from build123d import *

# Parameters (mm, degrees)
CUT_EXTRUDE1_DEPTH = 5
CUT_EXTRUDE2_DEPTH = 5


with BuildPart() as part:
    # Sketch1 → Revolve1 (revolve)
    with BuildSketch(Plane.XY, mode=Mode.PRIVATE) as revolve1_sk:
        Polygon((0, 0), (326, 0), (326, 16.5), (325, 17.5), (324, 17.5), (324, 16.1), (322.5, 16.1), (322.5, 17.5), (308.5, 17.5), (308.5, 20.5), (199.5, 20.5), (199.5, 17.5), (101.5, 17.5), (101.5, 16.1), (100, 16.1), (100, 17.5), (1, 17.5), (0, 16.5), align=None)
    revolve(revolve1_sk.sketch.rotate(Axis((0, 0, 0), (1, 0, 0)), 90), axis=Axis((0, 0, 0), (1, 0, 0)))

    # Sketch2 → Cut-Extrude1 (cut)
    with BuildSketch(Plane(origin=(0, 17.5, 0), x_dir=(1, 0, 0), z_dir=(0, 1, 0))):
        with BuildLine():
            Line((189.5, -5), (149.5, -5))
            ThreePointArc((149.5, -5), (144.5, 0), (149.5, 5))
            Line((149.5, 5), (189.5, 5))
            ThreePointArc((189.5, 5), (194.5, 0), (189.5, -5))
        make_face()
    extrude(amount=-CUT_EXTRUDE1_DEPTH, mode=Mode.SUBTRACT)

    # Sketch3 → Cut-Extrude2 (cut)
    with BuildSketch(Plane(origin=(0, 17.5, 0), x_dir=(1, 0, 0), z_dir=(0, 1, 0))):
        with BuildLine():
            Line((189.5, 5), (149.5, 5))
            ThreePointArc((149.5, 5), (144.5, 0), (149.5, -5))
            Line((149.5, -5), (189.5, -5))
            ThreePointArc((189.5, -5), (194.5, 0), (189.5, 5))
        make_face()
        with BuildLine():
            Line((10, 5), (50, 5))
            ThreePointArc((50, 5), (55, 0), (50, -5))
            Line((50, -5), (10, -5))
            ThreePointArc((10, -5), (5, 0), (10, 5))
        make_face()
    extrude(amount=-CUT_EXTRUDE2_DEPTH, mode=Mode.SUBTRACT)


solid = part.part
Verification items for the finished model (mm, model axes). A direction names the side the tool comes from. Round coordinates to 2 decimals unless told otherwise and drop trailing zeros. Loops run counter-clockwise (first coordinate to the right, second up) from the corner with the lowest first, then second, coordinate; pieces in that order, holes last. Notation, with made-up numbers: (54, -1.75) - (78, -1.75) arc R7 ccw to (78, 6.25) - close; hole circle Ø2 at (-5.75, -20.75). An arc over 180 degrees is marked (long way). Write item = value, one per line.
Q1. Material ranges on L1, parallel to X at y = -5.5, z = -16; L2, parallel to X at y = -12.5, z = 11; L3, parallel to X at y = -9.5, z = 15, recorded low to high.
Here are the results:
L1 = 0.42 to 100, 101.5 to 322.5, 324 to 325.58
L2 = 0.15 to 100, 101.5 to 322.5, 324 to 325.85
L3 = 199.5 to 308.5
Q2. Sectioned sample at D-D on x = 210. Record the boundary of the cut face in (y, z), plus the area to 3 significant figures.
Here are the results:
outline = circle Ø41 at (0, 0)
area = 1,320 mm^2
Q3. Depth check by flat-ended pin: pin 1 (4.5 mm diameter, centred on x = 37, y = 15, fed in from -Z); pin 2 (12 mm diameter, centred on x = 84, y = 4, fed in from -Z); pin 3 (3.5 mm diameter, centred on x = 38, y = 13.5, fed in from +Z); pin 4 (1 mm diameter, centred on y = 15.5, z = 0.5, fed in from -X). Enter the tip coordinate at first touch or a pass-through.
Here are the results:
pin_1 = -11.99
pin_2 = -17.5
pin_3 = 12.97
pin_4 = 0
Q4. Tool access check on faces 4 (the cylindrical face through (149.814, -14.756, 9.408)), 5 (the flat face through (322.5, 5.1, -15.5)), 6 (the flat face through (170, 12.5, 0)). Record the directions out of +Z, -Z, +X, -X, +Y, -Y that give a thin tool (end or side, any length) a straight path to the whole face; none if there is none.
Here are the results:
face_4 = -X
face_5 = none
face_6 = +Y
Q5. Mould release check, pull along X, two halves, no side actions. Record for faces 1 (the flat face through (199.5, -9.2, 15.1)), 2 (the flat face through (308.5, -9.2, -15.1)), 3 (the cylindrical face through (100.74, -4.836, 15.357)): +X half, -X half, draft (parallel to the pull), parting line (faces both ways), or undercut.
Here are the results:
face_1 = -X half
face_2 = +X half
face_3 = undercut
Q6. Sectioned sample at B-B on x = 20. Record the boundary of the cut face in (y, z), plus the area to 3 significant figures.
Here are the results:
outline = (12.5, -5) - (12.5, 5) - (16.77, 5) arc R17.5 ccw (long way) to (16.77, -5) - close
area = 915 mm^2
Q7. Sectioned sample at C-C on x = 61.5. Record the boundary of the cut face in (y, z).
Here are the results:
outline = circle Ø35 at (0, 0)
